Study the drawing (mm; zero at the part's minimum x, y, z) and answer. Coordinates: 2 decimals unless noted, no trailing zeros. Order: outer loops, then holes, each group sorted by start corner. A loop starts at its lowest first (then second) coordinate and runs counter-clockwise, first axis right, second up.
1. The part is cut by section B-B, the plane z = 1.25. Give the vertices of the cut face in (x, y), then the cut area to 3 significant figures.
2. The part is cut by section C-C, the plane z = 9. Give the vertices of the cut face in (x, y), then the cut area to 3 significant figures.
3. A flat-ended cylindrical pin translates along its axis: pin 1 Ø3 at (x, z) = (9, 4.5) entering from +Y. Find the tip coordinate at first contact, or state that the pin passes through.
4. Find the intervals of material crossed by probe 1 along Y at (x, z) = (20.5, 2); probe 2 along Z at (x, y) = (18, 41.5); probe 3 along Y at (x, z) = (16, 7.75) (1 decimal), in increasing order.
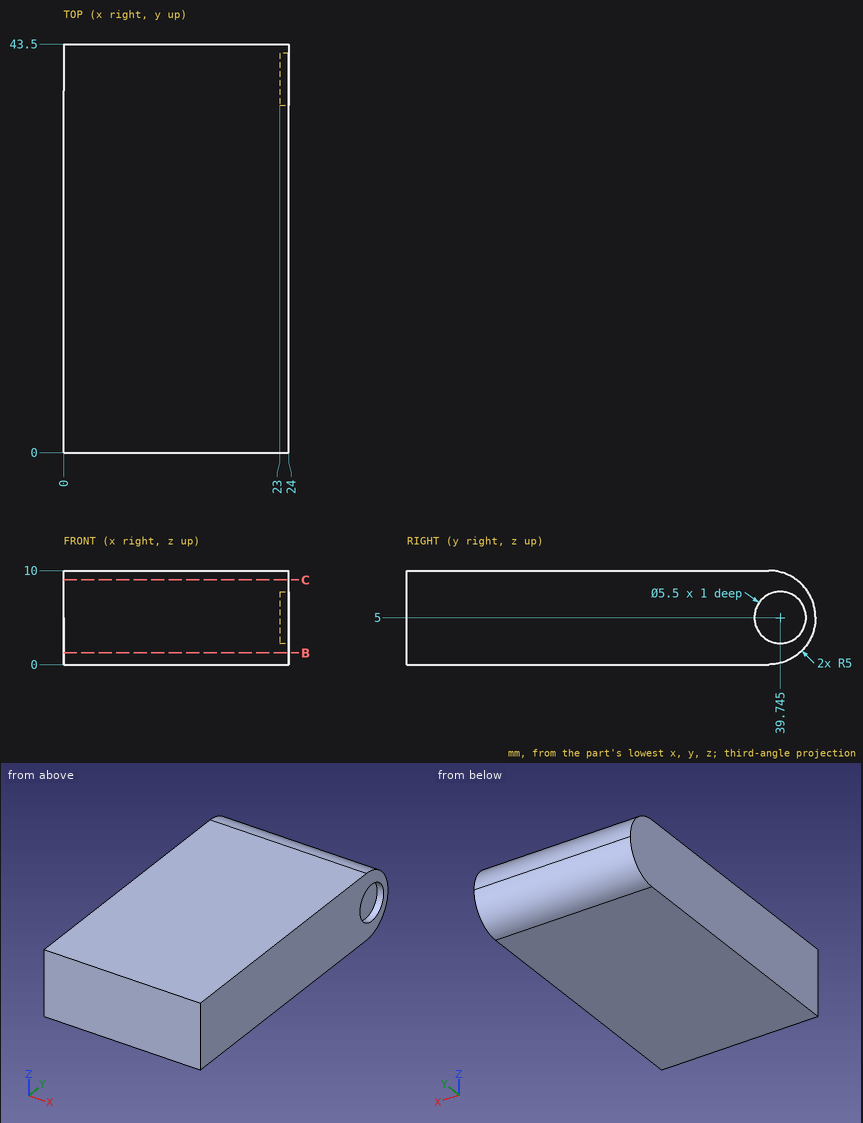
Geometry says:
1. outline: (0, 0) - (24, 0) - (24, 41.81) - (0, 41.81) - close
1. area: 1,000 mm2
2. outline: (0, 0) - (24, 0) - (24, 41.5) - (0, 41.5) - close
2. area: 996 mm2
3. pin 1: stops at y = 43.5
4. probe 1: y = 0 to 42.5
4. probe 2: z = 1 to 9
4. probe 3: y = 0 to 42.7
